```python
from build123d import *

# Parameters (mm, degrees)
F1_DEPTH = 254
F2_W     = 215.9
F2_H     = 92.64379
F2_H_2   = 91.50621
F3_DEPTH = 304.801
F5_DEPTH = 111.69479
F7_DEPTH = 111.69479


with BuildPart() as f1:
    # F0 (on Right) → F1 (new body)
    with BuildSketch(Plane.YZ):
        Polygon((25.96879, 119.263514), (-24.83121, 119.263514), (-101.03121, -109.336486), (-101.03121, -185.536486), (102.16879, -185.536486), (102.16879, -109.336486), align=None)
    extrude(amount=F1_DEPTH)

    # F2 (on face) → F3 (cut, through all)
    with BuildSketch(Plane.XY.offset(119.263514)):
        with Locations((127, 55.846895)):
            Rectangle(F2_W, F2_H)
        with Locations((127, -55.278105)):
            Rectangle(F2_W, F2_H_2)
    extrude(amount=-F3_DEPTH, mode=Mode.SUBTRACT)

    # F4 (on face) → F5 (cut, through all)
    with BuildSketch(Plane.XZ.offset(9.525)):
        with BuildLine():
            Line((184.15, 87.513514), (69.85, 87.513514))
            ThreePointArc((69.85, 87.513514), (60.869744, 83.79377), (57.15, 74.813514))
            Line((57.15, 74.813514), (57.15, -141.086486))
            ThreePointArc((57.15, -141.086486), (60.869744, -150.066742), (69.85, -153.786486))
            Line((69.85, -153.786486), (184.15, -153.786486))
            ThreePointArc((184.15, -153.786486), (193.130256, -150.066742), (196.85, -141.086486))
            Line((196.85, -141.086486), (196.85, 74.813514))
            ThreePointArc((196.85, 74.813514), (193.130256, 83.79377), (184.15, 87.513514))
        make_face()
    extrude(amount=-F5_DEPTH, mode=Mode.SUBTRACT)

    # F6 (on face) → F7 (cut, through all)
    with BuildSketch(Plane.XZ.offset(9.525)):
        with BuildLine():
            ThreePointArc((38.1, 87.513514), (35.854936, 86.583578), (34.925, 84.338514))
            Line((34.925, 84.338514), (34.925, -150.611486))
            ThreePointArc((34.925, -150.611486), (35.854936, -152.85655), (38.1, -153.786486))
            ThreePointArc((38.1, -153.786486), (40.345064, -152.85655), (41.275, -150.611486))
            Line((41.275, -150.611486), (41.275, 84.338514))
            ThreePointArc((41.275, 84.338514), (40.345064, 86.583578), (38.1, 87.513514))
        make_face()
        with BuildLine():
            ThreePointArc((215.9, -153.786486), (218.145064, -152.85655), (219.075, -150.611486))
            Line((219.075, -150.611486), (219.075, 84.338514))
            ThreePointArc((219.075, 84.338514), (218.145064, 86.583578), (215.9, 87.513514))
            ThreePointArc((215.9, 87.513514), (213.654936, 86.583578), (212.725, 84.338514))
            Line((212.725, 84.338514), (212.725, -150.611486))
            ThreePointArc((212.725, -150.611486), (213.654936, -152.85655), (215.9, -153.786486))
        make_face()
    extrude(amount=-F7_DEPTH, mode=Mode.SUBTRACT)


solid = f1.part
```
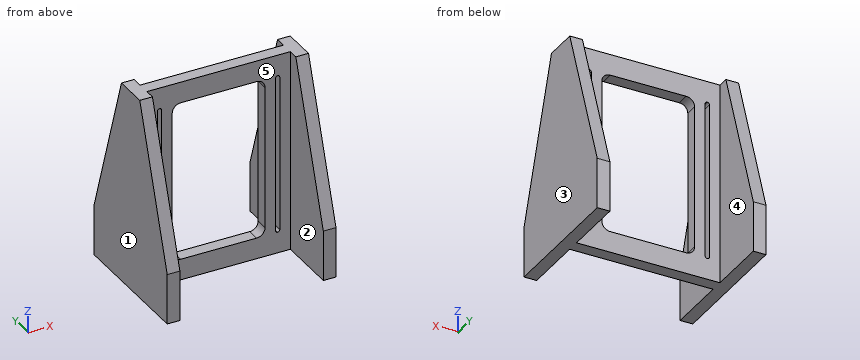
Can you work these out from the model? Positions are in its coordinate system, mm. Face numbers are marked on the shaded views. A direction names the side the tool comes from. Give positions to 0.01 mm unless a question says otherwise; leave off trailing zeros. Order: outer loops, then holes, each group sorted by start corner. A loop starts at its lowest first (then second) coordinate and runs counter-clockwise, first axis right, second up. Notation, with made-up numbers: (50.25, 49) - (93.25, 49) arc R20 ccw to (93.25, 86) - close; hole circle Ø5 at (39, -7). An arc over 180 degrees is marked (long way). Use a Markdown table: item, result. Add a question column.
Q1. If we section it at B-B on y = -20.5: Write out the boundary of the cut face in (x, z).
Q2. If we section it at D-D on z = -101.5: Write out the boundary of the cut face in (x, y) (3 decimals), plus the area to 3 significant figures.
Q3. If we mould it in two halves opening along X, with no side actions, what happens to the marked faces 1, 2 and 3? For each: released by +X, released by -X, zero draft, split by the parting line, or undercut.
Q4. Please list where these lines run through material, in increasing order: line 1 along Z through (x, y) = (105, -6); line 2 along X through (y, z) = (4.5, 25) (3 decimals); line 3 along X through (y, z) = (-87.5, -148).
Q5. If we section it at C-C on z = -60: Write out the boundary of the cut face in (x, y) (3 decimals), plus the area to 3 significant figures.
Q6. On a 3-axis mill with a long thin cutter (end or side, diameter ignored), from which of +Z, -Z, +X, -X, +Y, -Y can I reach the whole of each face in a straight line? I mean the marked faces 4 and 5. Say none if no direction works.
Q7. If we section it at A-A on x = 89.5: Write out the boundary of the cut face in (y, z) (3 decimals), plus the area to 3 significant figures.
Q8. I'm going to push flat-ended pins straight in: pin 1 (4 mm diameter, centred on x = 62.5, z = 83, fed in from +Y) (3 decimals); pin 2 (8 mm diameter, centred on x = 51.5, z = -8, fed in from -Y) (3 decimals). Where does each tip first touch, or does it pass through?
Answers follow:
| question | item | result |
|---|---|---|
| 1 | outline | (0, -185.54) - (19.05, -185.54) - (19.05, 119.26) - (0, 119.26) - close; (234.95, -185.54) - (254, -185.54) - (254, 119.26) - (234.95, 119.26) - close |
| 2 | outline | (0, -98.419) - (19.05, -98.419) - (19.05, -9.525) - (34.925, -9.525) - (34.925, 9.525) - (19.05, 9.525) - (19.05, 99.557) - (0, 99.557) - close; (41.275, -9.525) - (57.15, -9.525) - (57.15, 9.525) - (41.275, 9.525) - close; (196.85, -9.525) - (212.725, -9.525) - (212.725, 9.525) - (196.85, 9.525) - close; (219.075, -9.525) - (234.95, -9.525) - (234.95, -98.419) - (254, -98.419) - (254, 99.557) - (234.95, 99.557) - (234.95, 9.525) - (219.075, 9.525) - close |
| 2 | area | 8,750 mm^2 |
| 3 | face 1 | released by -X |
| 3 | face 2 | undercut |
| 3 | face 3 | released by +X |
| 4 | line 1 | z = -185.54 to -153.79, 87.51 to 119.26 |
| 4 | line 2 | x = 0 to 34.925, 41.275 to 57.15, 196.85 to 212.725, 219.075 to 254 |
| 4 | line 3 | x = 0 to 19.05, 234.95 to 254 |
| 5 | outline | (0, -84.586) - (19.05, -84.586) - (19.05, -9.525) - (34.925, -9.525) - (34.925, 9.525) - (19.05, 9.525) - (19.05, 85.723) - (0, 85.723) - close; (41.275, -9.525) - (57.15, -9.525) - (57.15, 9.525) - (41.275, 9.525) - close; (196.85, -9.525) - (212.725, -9.525) - (212.725, 9.525) - (196.85, 9.525) - close; (219.075, -9.525) - (234.95, -9.525) - (234.95, -84.586) - (254, -84.586) - (254, 85.723) - (234.95, 85.723) - (234.95, 9.525) - (219.075, 9.525) - close |
| 5 | area | 7,700 mm^2 |
| 6 | face 4 | +Z, -Z, +Y |
| 6 | face 5 | +Z, -Z, -Y |
| 7 | outline | (-9.525, -185.536) - (9.525, -185.536) - (9.525, -153.786) - (-9.525, -153.786) - close; (-9.525, 87.514) - (9.525, 87.514) - (9.525, 119.264) - (-9.525, 119.264) - close |
| 7 | area | 1,210 mm^2 |
| 8 | pin 1 | stops at y = 9.525 |
| 8 | pin 2 | stops at y = -9.525 |
